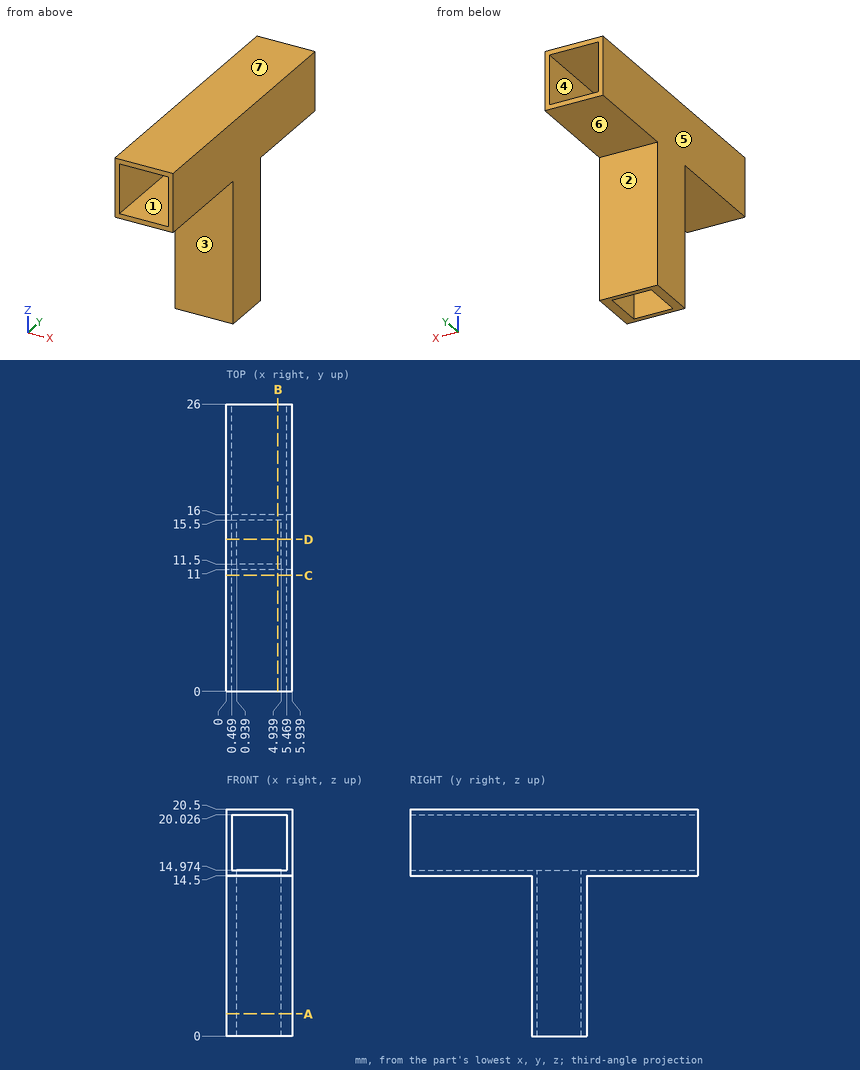
Print and shaded views of the part. All mm, measured from the part's lowest x, y and z. A direction names the side the tool comes from. Give positions to 0.01 mm unless a question says otherwise; leave off trailing zeros. Loops run counter-clockwise (first coordinate to the right, second up) from the corner with the lowest first, then second, coordinate; pieces in that order, holes last. Notation, with made-up numbers: (84, -0.5) - (112, -0.5) arc R9 ccw to (112, 14.5) - close; hole circle Ø2 at (39, -17). An arc over 180 degrees is marked (long way). Use a Markdown table: item, result.
(1) Wall check: line 1 along Z through (x, y) = (4.75, 21.75); line 2 along X through (y, z) = (3.75, 19.75); line 3 along Y through (x, z) = (2.75, 1.75). Give the ranges that are in metal, low to high.
Taken from the geometry:
| item | result |
|---|---|
| line 1 | 14.5 to 14.97, 20.03 to 20.5 |
| line 2 | 0 to 0.47, 5.47 to 5.94 |
| line 3 | 11 to 11.5, 15.5 to 16 |
(2) Band-saw the part on C-C (y = 10.5). Give the cut face in (x, z).
Taken from the geometry:
| item | result |
|---|---|
| outline | (0, 14.5) - (5.94, 14.5) - (5.94, 20.5) - (0, 20.5) - close; hole (0.47, 14.97) - (5.47, 14.97) - (5.47, 20.03) - (0.47, 20.03) - close |
(3) Band-saw the part on B-B (x = 4.65). Give the cut face in (y, z).
Taken from the geometry:
| item | result |
|---|---|
| outline | (0, 14.5) - (11, 14.5) - (11, 0) - (11.5, 0) - (11.5, 14.97) - (0, 14.97) - close; (0, 20.03) - (26, 20.03) - (26, 20.5) - (0, 20.5) - close; (15.5, 0) - (16, 0) - (16, 14.5) - (26, 14.5) - (26, 14.97) - (15.5, 14.97) - close |
(4) Drop flat-ended pins along their axis: pin 1 Ø3 at (x, y) = (3.5, 5.5) entering from -Z; pin 2 Ø3 at (x, z) = (3.5, 6) entering from -Y. Give the stop position or say it passes through.
Taken from the geometry:
| item | result |
|---|---|
| pin 1 | z = 14.5 |
| pin 2 | y = 11 |
(5) Band-saw the part on D-D (y = 13.75). Give the cut face in (x, z).
Taken from the geometry:
| item | result |
|---|---|
| outline | (0, 0) - (0.94, 0) - (0.94, 14.97) - (0.47, 14.97) - (0.47, 20.03) - (5.47, 20.03) - (5.47, 14.97) - (4.94, 14.97) - (4.94, 0) - (5.94, 0) - (5.94, 20.5) - (0, 20.5) - close |
(6) Which spindle directions (+Z, -Z, +X, -X, +Y, -Y) get a long thin tool onto all of the face, cutting with end or side? Do the marked faces 1, 2 and 3. Say none if no direction does.
Taken from the geometry:
| item | result |
|---|---|
| face 1 | +Y, -Y |
| face 2 | -Z, +X, -X, +Y |
| face 3 | -Z, +X, -X, -Y |
(7) Pull direction Z, two halves, no side cores. Call the marked faces 4, 5, 6 and 7: +Z half, -Z half, draft (parallel to the pull), parting line (faces both ways), or undercut.
Taken from the geometry:
| item | result |
|---|---|
| face 4 | undercut |
| face 5 | draft |
| face 6 | -Z half |
| face 7 | +Z half |
(8) Band-saw the part on A-A (z = 2). Give the cut face in (x, y), and give its area (3 significant figures).
Taken from the geometry:
| item | result |
|---|---|
| outline | (0, 11) - (5.94, 11) - (5.94, 16) - (0, 16) - close; hole (0.94, 11.5) - (4.94, 11.5) - (4.94, 15.5) - (0.94, 15.5) - close |
| area | 13.7 mm2 |
